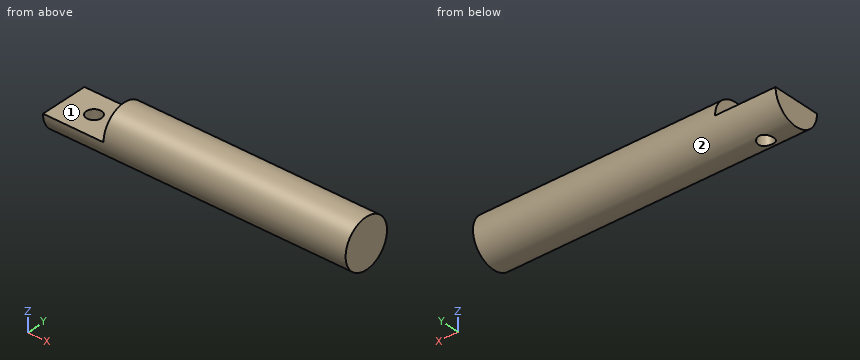
```python
from build123d import *

# Parameters (mm, degrees)
F0_R     = 4
F1_DEPTH = 40
F3_DEPTH = 10
F5_D     = 2.5


with BuildPart() as f1:
    # F0 (on Right) → F1 (new body)
    with BuildSketch(Plane.YZ):
        Circle(F0_R)
    extrude(amount=F1_DEPTH)

    # F2 (on face) → F3 (join)
    with BuildSketch(Plane(origin=(0, 0, 0), x_dir=(0, -1, 0), z_dir=(-1, 0, 0))):
        with BuildLine():
            Line((4, 0), (-4, 0))
            ThreePointArc((-4, 0), (0, -4), (4, 0))
        make_face()
    extrude(amount=F3_DEPTH)

    # F5 (through all)
    with Locations(Plane.XY):
        with Locations((-5, 0)):
            Hole(F5_D / 2)


solid = f1.part
```
Verification items for the finished model (mm, model axes). Face numbers are marked on the shaded views. A direction names the side the tool comes from. Coordinates: 2 decimals unless noted, no trailing zeros. Write each loop counter-clockwise with the first axis right and the second up, starting at its lowest first coordinate (ties: lowest second). Pieces come first, ordered by that corner, then holes. Notation, with made-up numbers: M -33.75,66.5 L -7.75,66.5 A22 ccw -7.75,80.5 Z; hole C -19.5,86 d7. An arc over 180 degrees is marked long. Answer as a JSON object with one key per item and string values. Group by question number.
(1) Cross-section at D-D, the plane y = -3. Record the cut outline in (x, z), and give its area (3 significant figures).
(2) Cross-section at C-C, the plane z = -3. Record the cut outline in (x, y), and give its area (3 significant figures).
(3) Cross-section at B-B, the plane x = -1. Record the cut outline in (y, z), and give its area (3 significant figures).
(4) Cross-section at A-A, the plane y = 0. Record the cut outline in (x, z).
(5) Tool access check on the marked faces 1 and 2. Record the directions out of +Z, -Z, +X, -X, +Y, -Y that give a thin tool (end or side, any length) a straight path to the whole face; none if there is none.
(6) Material ranges on line 1 (X direction, y = 0, z = -3.15); line 2 (Y direction, x = -5, z = -2.1); line 3 (Y direction, x = -5, z = -2.75), recorded low to high.
(7) Gauge pin test, flat ends, axial feed: pin 1 (1.5 mm diameter, centred on x = 19, z = -1, fed in from -Y); pin 2 (1.5 mm diameter, centred on x = -0.5, y = -2.5, fed in from -Z); pin 3 (1 mm diameter, centred on x = 18.5, y = -3, fed in from -Z). Record the tip position at first contact, or that the pin passes through.
Reply:
{
 "1": {"outline": "M -10,-2.65 L 40,-2.65 L 40,2.65 L 0,2.65 L 0,0 L -10,0 Z", "area": "238 mm²"},
 "2": {"outline": "M -10,-2.65 L 40,-2.65 L 40,2.65 L -10,2.65 Z; hole C -5,0 d2.5", "area": "260 mm²"},
 "3": {"outline": "M -4,0 A4 ccw 4,0 Z", "area": "25.1 mm²"},
 "4": {"outline": "M -10,-4 L -6.25,-4 L -6.25,0 L -10,0 Z; M -3.75,-4 L 40,-4 L 40,4 L 0,4 L 0,0 L -3.75,0 Z"},
 "5": {"face 1": "+Z, -X, +Y, -Y", "face 2": "+X, -X"},
 "6": {"line 1": "-10 to -6.25, -3.75 to 40", "line 2": "-3.4 to -1.25, 1.25 to 3.4", "line 3": "-2.9 to -1.25, 1.25 to 2.9"},
 "7": {"pin 1": "y = -3.99", "pin 2": "z = -3.6", "pin 3": "z = -3.12"}
}
